Source: CAD feature listing. Evaluate the final solid. Frame: model axes, mm. Face numbers are marked on the shaded views. A direction names the side the tool comes from. Round coordinates to 2 decimals unless told otherwise and drop trailing zeros. Loops run counter-clockwise (first coordinate to the right, second up) from the corner with the lowest first, then second, coordinate; pieces in that order, holes last. Notation, with made-up numbers: (86, 10) -> (94, 10) arc R15 ccw to (94, 29) -> close; hole circle Ø3 at (-12.5, 69). An arc over 180 degrees is marked (long way). Return JSON: item names as keys, results as strings. Group by question number.
```python
from build123d import *

# Parameters (mm, degrees)
SKETCH1_R           = 35
BOSS_EXTRUDE1_DEPTH = 150
CUT_EXTRUDE1_START  = -10
SKETCH3_R           = 34
CUT_EXTRUDE1_DEPTH  = 10


with BuildPart() as part:
    # Sketch1 → Boss-Extrude1 (new body)
    with BuildSketch(Plane(origin=(0, 0, 0), x_dir=(1, 0, 0), z_dir=(0, 1, 0))):
        with Locations(Location((0, 0, 0), (0, 0, 270))):
            Circle(SKETCH1_R)
        with BuildLine():
            Line((-31.448370387, -10), (31.448370387, -10))
            ThreePointArc((31.448370387, -10), (0, 33), (-31.448370387, -10))
        make_face(mode=Mode.SUBTRACT)
        with BuildLine():
            Line((-30.740852298, -12), (30.740852298, -12))
            ThreePointArc((30.740852298, -12), (0, -33), (-30.740852298, -12))
        make_face(mode=Mode.SUBTRACT)
    extrude(amount=BOSS_EXTRUDE1_DEPTH)

    # Sketch3 → Cut-Extrude1 (cut)
    with BuildSketch(Plane(origin=(0, 150, 0), x_dir=(1, 0, 0), z_dir=(0, 1, 0)).offset(CUT_EXTRUDE1_START)):
        with Locations(Location((0, 0, 0), (0, 0, 270))):
            Circle(SKETCH3_R)
        with BuildLine():
            Line((31.112698372, -11), (-31.112698372, -11))
            ThreePointArc((-31.112698372, -11), (0, 33), (31.112698372, -11))
        make_face(mode=Mode.SUBTRACT)
        with BuildLine():
            Line((-30.740852298, -12), (30.740852298, -12))
            ThreePointArc((30.740852298, -12), (0, -33), (-30.740852298, -12))
        make_face(mode=Mode.SUBTRACT)
    extrude(amount=CUT_EXTRUDE1_DEPTH, mode=Mode.SUBTRACT)


solid = part.part
```
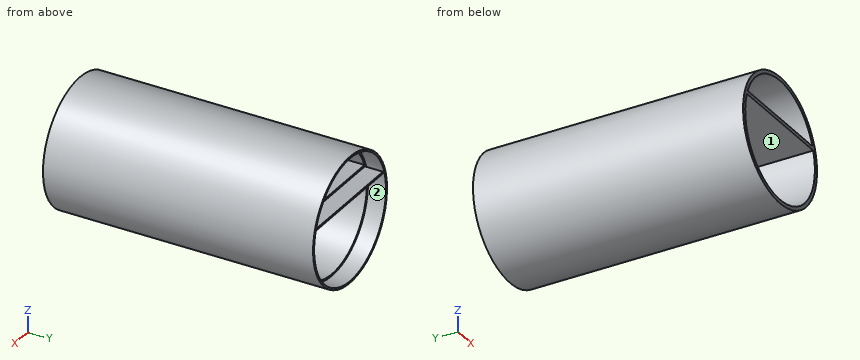
(1) Cut plane A-A (x = 0). Return loops of the section in (y, z).
(2) Cut plane B-B (z = 0). Return loops of the section in (x, y), and give its area (3 significant figures).
(3) Cut plane D-D (z = 23.5). Return loops of the section in (x, y).
(4) Ray query, line 1 (Z direction, x = -1, y = 127.5); line 2 (Z direction, x = 22, y = 128); line 3 (X direction, y = 143, z = 0). Return the intervals inside material, ascending.
(5) Cut plane C-C (y = 48.5). Return loops of the section in (x, z), and give its area (3 significant figures).
(6) Pin query (flat end, axial travel): pin 1 (12 mm diameter, centred on x = 10.5, y = 57.5, fed in from +Z); pin 2 (2 mm diameter, centred on x = -19, y = 62.5, fed in from -Z); pin 3 (6 mm diameter, centred on y = 66, z = -17.5, fed in from -X); pin 4 (8 mm diameter, centred on x = 8, z = 25.5, fed in from -Y). Return the tip coordinate at first contact, or that it passes through.
(7) Set-up query: the marked faces 1 and 2. Return all of +Z, -Z, +X, -X, +Y, -Y with unobstructed straight access to the full face (end or side cutting, diameter ignored); none if empty.
Answers follow:
{
 "1": {"outline": "(0, -35) -> (150, -35) -> (150, -34) -> (140, -34) -> (140, -33) -> (0, -33) -> close; (0, 10) -> (150, 10) -> (150, 11) -> (140, 11) -> (140, 12) -> (0, 12) -> close; (0, 33) -> (140, 33) -> (140, 34) -> (150, 34) -> (150, 35) -> (0, 35) -> close"},
 "2": {"outline": "(-35, 0) -> (-33, 0) -> (-33, 140) -> (-34, 140) -> (-34, 150) -> (-35, 150) -> close; (33, 0) -> (35, 0) -> (35, 150) -> (34, 150) -> (34, 140) -> (33, 140) -> close", "area": "580 mm^2"},
 "3": {"outline": "(-25.94, 0) -> (-23.17, 0) -> (-23.17, 140) -> (-24.57, 140) -> (-24.57, 150) -> (-25.94, 150) -> close; (23.17, 0) -> (25.94, 0) -> (25.94, 150) -> (24.57, 150) -> (24.57, 140) -> (23.17, 140) -> close"},
 "4": {"line 1": "-34.99 to -32.98, 10 to 12, 32.98 to 34.99", "line 2": "-27.22 to -24.6, 10 to 12, 24.6 to 27.22", "line 3": "-35 to -34, 34 to 35"},
 "5": {"outline": "circle Ø70 at (0, 0); hole (-31.45, 10) arc R33 ccw (long way) to (31.45, 10) -> close; hole (-30.74, 12) -> (30.74, 12) arc R33 ccw to start", "area": "552 mm^2"},
 "6": {"pin 1": "z = 34.71", "pin 2": "z = -30.02", "pin 3": "x = -31.86", "pin 4": "through"},
 "7": {"face 1": "+Y, -Y", "face 2": "+Y"}
}
